Build history of the part. All positions in model axes, mm. Give positions to 0.01 mm unless a question says otherwise; leave off trailing zeros. Loops run counter-clockwise (first coordinate to the right, second up) from the corner with the lowest first, then second, coordinate; pieces in that order, holes last. Notation, with made-up numbers: (73.25, 27.5) -> (127.25, 27.5) arc R14 cw to (127.25, 52.5) -> close; hole circle Ø5 at (82, 49.25). An arc over 180 degrees is marked (long way). One line per question, with ' | ' between items. Start each with the question number.
(1) Slice it at C-C, the plane z = 2.5. Give the number of separate pieces and of enclosed holes in the cut face, then the cut area to 3 significant figures.
(2) Slice it at A-A, the plane y = 67. Write the cut outline in (x, z), then the cut area to 3 significant figures.
(3) Slice it at B-B, the plane x = 82.5. Write the cut outline in (y, z).
(4) Drill centre lines: L1, parallel to Y at x = -74, z = 1.2; L2, parallel to X at y = 3.5, z = 2.55; L3, parallel to X at y = -59, z = 2.65. Where is each one in solid material? Low to high. Write a range as from..to.
(5) Flat gauge pin, fed straight in: pin 1 Ø7 at (x, y) = (-60, 60) entering from -Z. Where does the tip first touch, or does it go through?
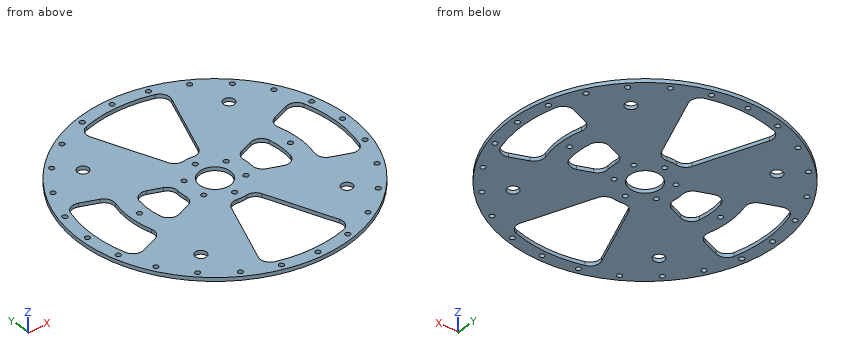
```python
from build123d import *

# Parameters (mm, degrees)
SKETCH_1_R      = 110
SKETCH_1_R_2    = 2
SKETCH_1_R_3    = 4.5
SKETCH_1_R_4    = 12.5
EXTRUDE_1_DEPTH = 3


with BuildPart() as part:
    # 草图1 → 凸台-拉伸1 (new body)
    with BuildSketch(Plane.XY):
        Circle(SKETCH_1_R)
        with Locations((-74.246212025, -74.246212025)):
            Circle(SKETCH_1_R_2, mode=Mode.SUBTRACT)
        with Locations((-60, -60)):
            Circle(SKETCH_1_R_3, mode=Mode.SUBTRACT)
        with Locations((-52.42, -90.794103333)):
            Circle(SKETCH_1_R_2, mode=Mode.SUBTRACT)
        with Locations((-27.175999736, -101.42221176)):
            Circle(SKETCH_1_R_2, mode=Mode.SUBTRACT)
        with Locations((-90.794103333, -52.42)):
            Circle(SKETCH_1_R_2, mode=Mode.SUBTRACT)
        with Locations((-101.42221176, -27.175999736)):
            Circle(SKETCH_1_R_2, mode=Mode.SUBTRACT)
        with Locations((-104.84, 0)):
            Circle(SKETCH_1_R_2, mode=Mode.SUBTRACT)
        with Locations((0, -20)):
            Circle(SKETCH_1_R_2, mode=Mode.SUBTRACT)
        with Locations((-17.320508076, -10)):
            Circle(SKETCH_1_R_2, mode=Mode.SUBTRACT)
        with Locations((0, -104.84)):
            Circle(SKETCH_1_R_2, mode=Mode.SUBTRACT)
        with Locations((27.175999736, -101.42221176)):
            Circle(SKETCH_1_R_2, mode=Mode.SUBTRACT)
        with Locations((52.42, -90.794103333)):
            Circle(SKETCH_1_R_2, mode=Mode.SUBTRACT)
        with BuildLine():
            ThreePointArc((3.969843853, -27.211952149), (9.14743169, -28.213122771), (12.577035349, -32.219065502))
            Line((12.577035349, -32.219065502), (33.327823236, -85.377140959))
            ThreePointArc((33.327823236, -85.377140959), (33.055374747, -91.814593053), (28.125538485, -95.963295509))
            ThreePointArc((28.125538485, -95.963295509), (0, -100), (-28.125538485, -95.963295509))
            ThreePointArc((-28.125538485, -95.963295509), (-33.055374747, -91.814593053), (-33.327823236, -85.377140959))
            Line((-33.327823236, -85.377140959), (-12.577035349, -32.219065502))
            ThreePointArc((-12.577035349, -32.219065502), (-9.14743169, -28.213122771), (-3.969843853, -27.211952149))
            ThreePointArc((-3.969843853, -27.211952149), (0, -27.5), (3.969843853, -27.211952149))
        make_face(mode=Mode.SUBTRACT)
        with Locations((74.246212025, -74.246212025)):
            Circle(SKETCH_1_R_2, mode=Mode.SUBTRACT)
        with Locations((60, -60)):
            Circle(SKETCH_1_R_3, mode=Mode.SUBTRACT)
        with Locations((17.320508076, -10)):
            Circle(SKETCH_1_R_2, mode=Mode.SUBTRACT)
        with Locations((90.794103333, -52.42)):
            Circle(SKETCH_1_R_2, mode=Mode.SUBTRACT)
        with Locations((101.42221176, -27.175999736)):
            Circle(SKETCH_1_R_2, mode=Mode.SUBTRACT)
        with BuildLine():
            Line((-71.806959395, -28.030566765), (-85.377140959, -33.327823236))
            ThreePointArc((-85.377140959, -33.327823236), (-91.814593053, -33.055374747), (-95.963295509, -28.125538485))
            ThreePointArc((-95.963295509, -28.125538485), (-100, 0), (-95.963295509, 28.125538485))
            ThreePointArc((-95.963295509, 28.125538485), (-91.814593053, 33.055374747), (-85.377140959, 33.327823236))
            Line((-85.377140959, 33.327823236), (-71.806959395, 28.030566765))
            ThreePointArc((-71.806959395, 28.030566765), (-67.565247924, 24.16516315), (-67.003234476, 18.453980943))
            ThreePointArc((-67.003234476, 18.453980943), (-69.49807798, 0), (-67.003234476, -18.453980943))
            ThreePointArc((-67.003234476, -18.453980943), (-67.565247924, -24.16516315), (-71.806959395, -28.030566765))
        make_face(mode=Mode.SUBTRACT)
        with Locations((-101.42221176, 27.175999736)):
            Circle(SKETCH_1_R_2, mode=Mode.SUBTRACT)
        with Locations((-62, 0)):
            Circle(SKETCH_1_R_2, mode=Mode.SUBTRACT)
        with Locations((-90.794103333, 52.42)):
            Circle(SKETCH_1_R_2, mode=Mode.SUBTRACT)
        with BuildLine():
            ThreePointArc((-27.211952149, -3.969843853), (-28.213122771, -9.14743169), (-32.219065502, -12.577035349))
            Line((-32.219065502, -12.577035349), (-42.670779868, -16.656966874))
            ThreePointArc((-42.670779868, -16.656966874), (-49.413037015, -16.226521741), (-53.421568975, -10.788232859))
            ThreePointArc((-53.421568975, -10.788232859), (-54.5, 0), (-53.421568975, 10.788232859))
            ThreePointArc((-53.421568975, 10.788232859), (-49.413037015, 16.226521741), (-42.670779868, 16.656966874))
            Line((-42.670779868, 16.656966874), (-32.219065502, 12.577035349))
            ThreePointArc((-32.219065502, 12.577035349), (-28.213122771, 9.14743169), (-27.211952149, 3.969843853))
            ThreePointArc((-27.211952149, 3.969843853), (-27.5, 0), (-27.211952149, -3.969843853))
        make_face(mode=Mode.SUBTRACT)
        with Locations((-17.320508076, 10)):
            Circle(SKETCH_1_R_2, mode=Mode.SUBTRACT)
        with Locations((-60, 60)):
            Circle(SKETCH_1_R_3, mode=Mode.SUBTRACT)
        with Locations((-74.246212025, 74.246212025)):
            Circle(SKETCH_1_R_2, mode=Mode.SUBTRACT)
        with Locations((-52.42, 90.794103333)):
            Circle(SKETCH_1_R_2, mode=Mode.SUBTRACT)
        with Locations((-27.175999736, 101.42221176)):
            Circle(SKETCH_1_R_2, mode=Mode.SUBTRACT)
        Circle(SKETCH_1_R_4, mode=Mode.SUBTRACT)
        with Locations((17.320508076, 10)):
            Circle(SKETCH_1_R_2, mode=Mode.SUBTRACT)
        with Locations((0, 20)):
            Circle(SKETCH_1_R_2, mode=Mode.SUBTRACT)
        with BuildLine():
            ThreePointArc((27.211952149, 3.969843853), (28.213122771, 9.14743169), (32.219065502, 12.577035349))
            Line((32.219065502, 12.577035349), (42.670779868, 16.656966874))
            ThreePointArc((42.670779868, 16.656966874), (49.413037015, 16.226521741), (53.421568975, 10.788232859))
            ThreePointArc((53.421568975, 10.788232859), (54.5, 0), (53.421568975, -10.788232859))
            ThreePointArc((53.421568975, -10.788232859), (49.413037015, -16.226521741), (42.670779868, -16.656966874))
            Line((42.670779868, -16.656966874), (32.219065502, -12.577035349))
            ThreePointArc((32.219065502, -12.577035349), (28.213122771, -9.14743169), (27.211952149, -3.969843853))
            ThreePointArc((27.211952149, -3.969843853), (27.5, 0), (27.211952149, 3.969843853))
        make_face(mode=Mode.SUBTRACT)
        with Locations((62, 0)):
            Circle(SKETCH_1_R_2, mode=Mode.SUBTRACT)
        with BuildLine():
            ThreePointArc((95.963295509, -28.125538485), (91.814593053, -33.055374747), (85.377140959, -33.327823236))
            Line((85.377140959, -33.327823236), (71.806959395, -28.030566765))
            ThreePointArc((71.806959395, -28.030566765), (67.565247924, -24.16516315), (67.003234476, -18.453980943))
            ThreePointArc((67.003234476, -18.453980943), (69.49807798, 0), (67.003234476, 18.453980943))
            ThreePointArc((67.003234476, 18.453980943), (67.565247924, 24.16516315), (71.806959395, 28.030566765))
            Line((71.806959395, 28.030566765), (85.377140959, 33.327823236))
            ThreePointArc((85.377140959, 33.327823236), (91.814593053, 33.055374747), (95.963295509, 28.125538485))
            ThreePointArc((95.963295509, 28.125538485), (100, 0), (95.963295509, -28.125538485))
        make_face(mode=Mode.SUBTRACT)
        with Locations((104.84, 0)):
            Circle(SKETCH_1_R_2, mode=Mode.SUBTRACT)
        with Locations((101.42221176, 27.175999736)):
            Circle(SKETCH_1_R_2, mode=Mode.SUBTRACT)
        with Locations((90.794103333, 52.42)):
            Circle(SKETCH_1_R_2, mode=Mode.SUBTRACT)
        with BuildLine():
            Line((33.327823236, 85.377140959), (12.577035349, 32.219065502))
            ThreePointArc((12.577035349, 32.219065502), (9.14743169, 28.213122771), (3.969843853, 27.211952149))
            ThreePointArc((3.969843853, 27.211952149), (0, 27.5), (-3.969843853, 27.211952149))
            ThreePointArc((-3.969843853, 27.211952149), (-9.14743169, 28.213122771), (-12.577035349, 32.219065502))
            Line((-12.577035349, 32.219065502), (-33.327823236, 85.377140959))
            ThreePointArc((-33.327823236, 85.377140959), (-33.055374747, 91.814593053), (-28.125538485, 95.963295509))
            ThreePointArc((-28.125538485, 95.963295509), (0, 100), (28.125538485, 95.963295509))
            ThreePointArc((28.125538485, 95.963295509), (33.055374747, 91.814593053), (33.327823236, 85.377140959))
        make_face(mode=Mode.SUBTRACT)
        with Locations((0, 104.84)):
            Circle(SKETCH_1_R_2, mode=Mode.SUBTRACT)
        with Locations((27.175999736, 101.42221176)):
            Circle(SKETCH_1_R_2, mode=Mode.SUBTRACT)
        with Locations((52.42, 90.794103333)):
            Circle(SKETCH_1_R_2, mode=Mode.SUBTRACT)
        with Locations((60, 60)):
            Circle(SKETCH_1_R_3, mode=Mode.SUBTRACT)
        with Locations((74.246212025, 74.246212025)):
            Circle(SKETCH_1_R_2, mode=Mode.SUBTRACT)
    extrude(amount=EXTRUDE_1_DEPTH)


solid = part.part
```
Final values:
1) separate pieces: 1 | enclosed holes: 43 | area: 24,800 mm2
2) outline: (-87.24, 0) -> (-26.15, 0) -> (-26.15, 3) -> (-87.24, 3) -> close; (26.15, 0) -> (87.24, 0) -> (87.24, 3) -> (26.15, 3) -> close | area: 367 mm2
3) outline: (-72.76, 0) -> (-32.2, 0) -> (-32.2, 3) -> (-72.76, 3) -> close; (32.2, 0) -> (72.76, 0) -> (72.76, 3) -> (32.2, 3) -> close
4) L1: -81.39..-76.23, -72.26..-28.89, 28.89..72.26, 76.23..81.39 | L2: -109.94..-99.94, -69.41..-54.39, -27.28..-12, 12..27.28, 54.39..69.41, 99.94..109.94 | L3: -92.84..-64.39, -55.61..-23.03, 23.03..55.61, 64.39..92.84
5) pin 1: through
